Can you work these out from the drawing? Everything is in mm from the part's minimum corner. A direction names the side the tool comes from. Round coordinates to 2 decimals unless told otherwise and drop trailing zeros. Loops run counter-clockwise (first coordinate to the right, second up) from the corner with the lowest first, then second, coordinate; pieces in that order, holes last. Notation, with made-up numbers: M -11,9 L -2,9 A15 cw -2,30 Z; hole C -10.5,30.25 d5. An arc over 180 degrees is marked long. Answer in a Markdown table with one row per item.
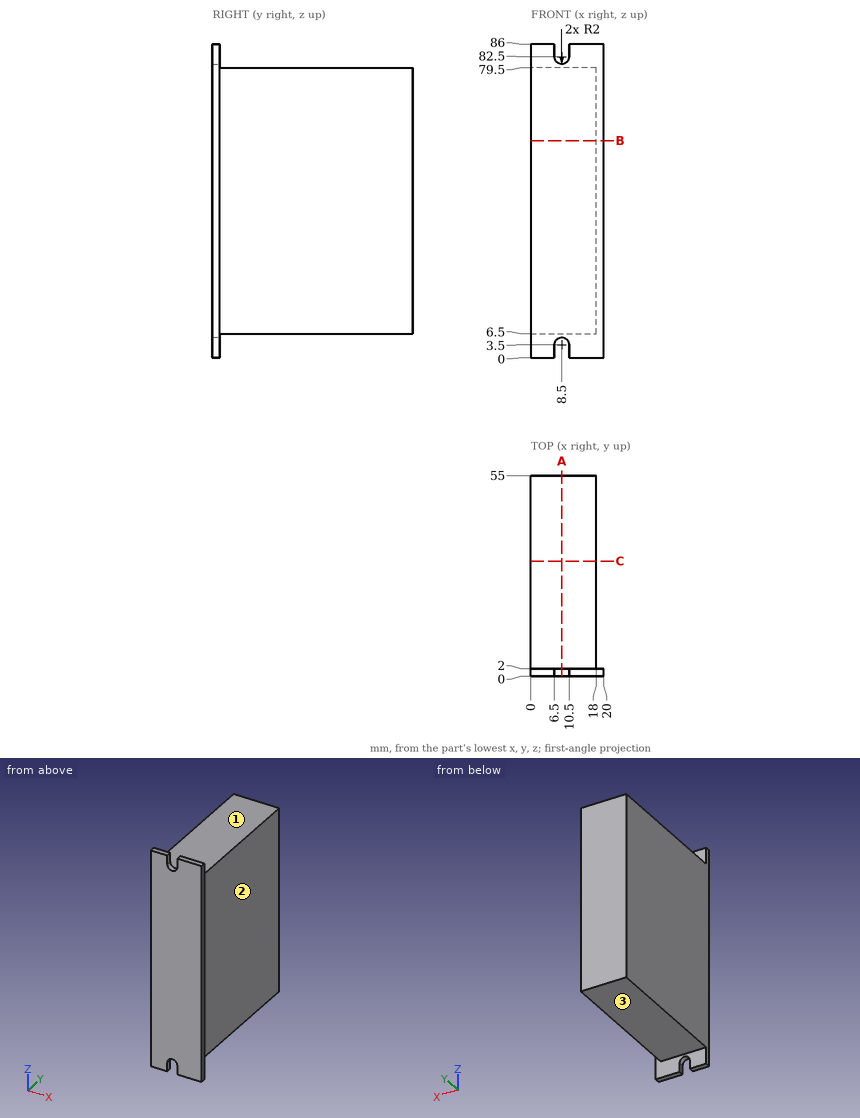
1) I need wall thicknesses on line 1 (Z direction, x = 13, y = 24.5); line 2 (X direction, y = 42, z = 70); line 3 (Y direction, x = 16.5, z = 5). Which ranges of each line are inside material? Lowest first, please.
Computed:
| item | result |
|---|---|
| line 1 | z = 6.5 to 79.5 |
| line 2 | x = 0 to 18 |
| line 3 | y = 0 to 2 |
2) I want a section at A-A, the plane x = 8.5. Please give me the cut outline in (y, z), plus the area to 3 significant figures.
Computed:
| item | result |
|---|---|
| outline | M 0,5.5 L 2,5.5 L 2,6.5 L 55,6.5 L 55,79.5 L 2,79.5 L 2,80.5 L 0,80.5 Z |
| area | 4,020 mm² |
3) Which directions (+Z, -Z, +X, -X, +Y, -Y) give clear straight access to the entire face, cutting with the end or side of a thin tool? Please do the marked faces 1, 2 and 3.
Computed:
| item | result |
|---|---|
| face 1 | +Z, +X, -X, +Y |
| face 2 | +Z, -Z, +X, +Y |
| face 3 | -Z, +X, -X, +Y |
4) Will these pins go through, and if not, where does the flat tip stop? P1, Ø6, axis at y = 34.5, z = 17, coming from the +X side; P2, Ø2, axis at x = 17, y = 14.5, coming from the -Z side; P3, Ø5.5, axis at x = 11, y = 41.5, coming from the +Z side.
Computed:
| item | result |
|---|---|
| P1 | stops at x = 18 |
| P2 | stops at z = 6.5 |
| P3 | stops at z = 79.5 |
5) I want a section at C-C, the plane y = 31.5. Please give me the cut outline in (x, z), plus the area to 3 significant figures.
Computed:
| item | result |
|---|---|
| outline | M 0,6.5 L 18,6.5 L 18,79.5 L 0,79.5 Z |
| area | 1,310 mm² |
6) I want a section at B-B, the plane z = 59.5. Please give me the cut outline in (x, y).
Computed:
| item | result |
|---|---|
| outline | M 0,0 L 20,0 L 20,2 L 18,2 L 18,55 L 0,55 Z |
